Part model, mm, in its own coordinate system. A direction names the side the tool comes from. Give positions to 0.01 mm unless a question says otherwise; leave off trailing zeros. Order: outer loops, then holes, each group sorted by start corner. A loop starts at its lowest first (then second) coordinate and runs counter-clockwise, first axis right, second up. Notation, with made-up numbers: (-33.75, 0) - (1.25, 0) arc R27 cw to (1.25, 25) - close; hole circle Ø8 at (61, -30.5). An arc over 180 degrees is marked (long way). One line per item, written item: value.
```python
from build123d import *

# Parameters (mm, degrees)
F0_R           = 38.1
F0_R_2         = 0.8751159205
F1_DEPTH       = 12.7
F2_R           = 9.525
F3_DEPTH       = 12.701
F4_R           = 12.7
F5_DEPTH       = 6.35
F7_D           = 3.175
F7_CBORE_D     = 6.35
F7_CBORE_DEPTH = 6.35
F8_R           = 23.8125
F8_R_2         = 22.225
F9_DEPTH       = 1.905


with BuildPart() as f1:
    # F0 (on Front) → F1 (new body)
    with BuildSketch(Plane.XZ):
        Circle(F0_R)
        with Locations((20.7111840319, 10.8808754866)):
            Circle(F0_R_2, mode=Mode.SUBTRACT)
        with Locations((20.7111840319, 10.8808754866)):
            Circle(F0_R_2)
    extrude(amount=F1_DEPTH)

    # F2 (on face) → F3 (cut, through all)
    with BuildSketch(Plane.XZ.offset(12.7)):
        Circle(F2_R)
    extrude(amount=-F3_DEPTH, mode=Mode.SUBTRACT)

    # F4 (on face) → F5 (cut)
    with BuildSketch(Plane.XZ.offset(12.7)):
        Circle(F4_R)
    extrude(amount=-F5_DEPTH, mode=Mode.SUBTRACT)

    # F7 (through all)
    with Locations(Plane.XZ.offset(12.7)):
        with Locations((0, 31.75), (31.75, 0), (0, -31.75), (-31.75, 0)):
            CounterBoreHole(F7_D / 2, F7_CBORE_D / 2, F7_CBORE_DEPTH)

    # F8 (on face) → F9 (cut)
    with BuildSketch(Plane(origin=(0, 0, 0), x_dir=(-1, 0, 0), z_dir=(0, 1, 0))):
        Circle(F8_R)
        Circle(F8_R_2, mode=Mode.SUBTRACT)
    extrude(amount=-F9_DEPTH, mode=Mode.SUBTRACT)


solid = f1.part
```
1) Which spindle directions (+Z, -Z, +X, -X, +Y, -Y) get a long thin tool onto all of the face, cutting with end or side? Do faces 1 (the cylindrical face through (-0.85, -3.13, 33.09)), 2 (the flat face through (20, -1.905, 11)), 3 (the flat face through (-30, -6.35, -1)). Say none if no direction does.
Outcome:
face 1: +Y, -Y
face 2: +Y
face 3: -Y
2) Cut at D-D, the plane z = 0. Give the number of separate pieces and of enclosed holes in the cut face, then the cut area to 3 significant figures.
Outcome:
separate pieces: 4
enclosed holes: 0
area: 558 mm^2
3) Mould opens along Z. For faces 4 (the cylindrical face through (18.897, -0.939, -14.49)), 5 (the flat face through (0, 0, -10)), 6 (the cylindrical face through (-30.235, -6.261, -23.183)) say: released by +Z, released by -Z, zero draft, split by the parting line, or undercut.
Outcome:
face 4: undercut
face 5: zero draft
face 6: split by the parting line
4) Cut at C-C, the plane y = -10.25. Give the cut face in (x, z) (3 decimals), then the cut area to 3 significant figures.
Outcome:
outline: circle Ø76.2 at (0, 0); hole circle Ø6.35 at (-31.75, 0); hole circle Ø25.4 at (0, 0); hole circle Ø6.35 at (0, -31.75); hole circle Ø6.35 at (0, 31.75); hole circle Ø6.35 at (31.75, 0)
area: 3,930 mm^2
5) Pin check, flat tips, straight feed: pin 1 (3 mm diameter, centred on x = -1, z = -31.5, fed in from -Y); pin 2 (6 mm diameter, centred on x = -25.5, y = -2, fed in from -Z); pin 3 (1.5 mm diameter, centred on x = 3.5, y = -6, fed in from +Z). Stop position of each tip, or through.
Outcome:
pin 1: stops at y = -6.35
pin 2: stops at z = -30.75
pin 3: stops at z = 38
6) Drill centre lines: line 1 along Z through (x, y) = (0, -0.85) (1 decimal); line 2 along Z through (x, y) = (0, -9) (3 decimals); line 3 along Z through (x, y) = (0, -2.75) (1 decimal). Where is each one in solid material? Low to high. Write a range as from..to.
Outcome:
line 1: z = -38.1..-33.3, -30.2..-23.8, -22.2..-9.5, 9.5..22.2, 23.8..30.2, 33.3..38.1
line 2: z = -38.1..-34.925, -28.575..-12.7, 12.7..28.575, 34.925..38.1
line 3: z = -38.1..-33.3, -30.2..-9.5, 9.5..30.2, 33.3..38.1
7) Cut at A-A, the plane z = 8. Give the cut face in (x, y) (3 decimals), then the cut area to 3 significant figures.
Outcome:
outline: (-37.251, -12.7) - (-9.864, -12.7) - (-9.864, -6.35) - (-5.17, -6.35) - (-5.17, 0) - (-20.735, 0) - (-20.735, -1.905) - (-22.428, -1.905) - (-22.428, 0) - (-37.251, 0) - close; (5.17, -6.35) - (9.864, -6.35) - (9.864, -12.7) - (37.251, -12.7) - (37.251, 0) - (22.428, 0) - (22.428, -1.905) - (20.735, -1.905) - (20.735, 0) - (5.17, 0) - close
area: 749 mm^2
